The listing builds one solid part. Answer for the finished solid, in the listing's coordinates (mm). A direction names the side the tool comes from. Round coordinates to 2 decimals unless told otherwise and drop trailing zeros. Order: outer loops, then holes, each group sorted by start corner. A loop starts at its lowest first (then second) coordinate and runs counter-clockwise, first axis right, second up. Notation, with made-up numbers: (72, 33) - (88, 33) arc R18 cw to (88, 48) - close; hole circle Ø2 at (60.25, 76.5). An arc over 180 degrees is marked (long way). Use CSV: the item, a comma, the result in double quotes. Start each with the question number.
Item 1: Find section B-B, the plane x = 43.5. Give the vertices of the cut face in (y, z).
Item 2: Flat-ended cylindrical pins translate along their axes: P1, Ø2.5, axis at x = 27.5, z = -15, coming from the +Y side; P2, Ø3.5, axis at x = 28.3, z = -17.12, coming from the -Y side; P3, Ø4, axis at y = 1.5, z = 2.5, coming from the +X side; P4, Ø1.5, axis at y = 2, z = 13.5, coming from the -X side. Find the tip coordinate at first contact, or state that the pin passes through.
Item 3: Find section A-A, the plane y = 4.75. Give the vertices of the cut face in (x, z).
Item 4: Determine the mould class of faces 1 (the flat face through (-49, 3.6, -21)), 2 (the cylindrical face through (42.228, 3.944, -8.156)), 3 (the flat face through (24, 3, 25.135)) for opening direction X: +X half, -X half, draft (parallel to the pull), parting line (faces both ways), or undercut.
Item 5: Straight lines are drawn through the part: line 1 along X through (y, z) = (4.75, -16); line 2 along X through (y, z) = (4.25, -20); line 3 along Z through (x, y) = (48, 5). For each, find the intervals that lie inside material, in ascending order. Write a range as [from, to].
Item 6: For faces 4 (the cylindrical face through (-54.776, 5.818, -19.497)), 5 (the cylindrical face through (24.024, 7.43, 24.534)), determine the directions among +Z, -Z, +X, -X, +Y, -Y from which every point of the face is accessible in a straight line to the end or side of a thin tool.
```python
from build123d import *

# Parameters (mm, degrees)
BOSS_EXTRUDE2_DEPTH                          = 8
CBORE_FOR_M4_HEX_SOCKET_HEAD_CAP_SCR_2_COUNT = 2
CBORE_FOR_M4_HEX_SOCKET_HEAD_CAP_SCR_2_PITCH = 43.312825964
CBORE_FOR_M4_HEX_SOCKET_HEAD_CAP_SCR_3_COUNT = 2
CBORE_FOR_M4_HEX_SOCKET_HEAD_CAP_SCR_3_PITCH = 79.131181871
FILLET1_R                                    = 2


with BuildPart() as part:
    # Sketch6 → Boss-Extrude2 (new body)
    with BuildSketch(Plane(origin=(0, 0, 0), x_dir=(1, 0, 0), z_dir=(0, 1, 0))):
        with BuildLine():
            Line((-49.241489328, 24.864510752), (-56.554028145, 24.864510752))
            ThreePointArc((-56.554028145, 24.864510752), (-41.909367204, -10.490828308), (-6.554028145, -25.135489248))
            Line((-6.554028145, -25.135489248), (55.470114159, -25.135489248))
            Line((55.470114159, -25.135489248), (55.470114159, -6.057055904))
            ThreePointArc((55.470114159, -6.057055904), (42.058086193, 8.373222092), (31.280664632, 24.864510752))
            Line((31.280664632, 24.864510752), (15.257491481, 24.864510752))
            Line((15.257491481, 24.864510752), (-49.241489328, 24.864510752))
        make_face()
    extrude(amount=BOSS_EXTRUDE2_DEPTH)

    # Sketch9 → CBORE for M4 Hex Socket Head Cap Screw1 (revolve, cut)
    with BuildSketch(Plane(origin=(28.299910658, 8, -17.122913845), x_dir=(0, 0, 1), z_dir=(1, 0, 0))):
        Polygon((0, 0), (0, 11.451936393), (2.25, 10.1), (2.25, 4.4), (4, 4.4), (4, 0.025), (4.025, 0), align=None)
    cbore_for_m4_hex_socket_head_cap_screw1 = revolve(axis=Axis((28.299910658, 14.35, -17.122913845), (0, -1, 0)), mode=Mode.SUBTRACT)

    # CBORE for M4 Hex Socket Head Cap Scr 2: CBORE for M4 Hex Socket Head Cap Screw1 ×2
    with Locations(*[Vector(0.5169167622472475, 0, 0.8560356656751065) * (i * CBORE_FOR_M4_HEX_SOCKET_HEAD_CAP_SCR_2_PITCH) for i in range(1, CBORE_FOR_M4_HEX_SOCKET_HEAD_CAP_SCR_2_COUNT)]):
        add(cbore_for_m4_hex_socket_head_cap_screw1, mode=Mode.SUBTRACT)

    # CBORE for M4 Hex Socket Head Cap Scr 3: CBORE for M4 Hex Socket Head Cap Screw1 ×2
    with Locations(*[Vector(-0.9997256378089421, 0, -0.023423259967479314) * (i * CBORE_FOR_M4_HEX_SOCKET_HEAD_CAP_SCR_3_PITCH) for i in range(1, CBORE_FOR_M4_HEX_SOCKET_HEAD_CAP_SCR_3_COUNT)]):
        add(cbore_for_m4_hex_socket_head_cap_screw1, mode=Mode.SUBTRACT)

    # Fillet1
    # the kernel refuses this fillet: 2 mm, written as the material it takes off along each edge
    with BuildSketch(Plane(origin=(-6.554028145, 8, -24.864510752), x_dir=(-0.99500015408545, 0, -0.09987338669500904), z_dir=(0.09987338669500904, 0, -0.99500015408545))) as fillet1_piece_1:
        with BuildLine():
            CenterArc((50 - FILLET1_R, -FILLET1_R), FILLET1_R, 0, 90)
            Line((50, -FILLET1_R), (50, 0))
            Line((50, 0), (50 - FILLET1_R, 0))
        make_face()
    revolve(axis=Axis((-6.554028145, 8, -24.864510752), (0, 1, 0)), revolution_arc=95.731879569, mode=Mode.SUBTRACT)
    with BuildSketch(Plane(origin=(-6.554028145, 8, 25.135489248), x_dir=(0, 0, -1), z_dir=(1, 0, 0))) as fillet1_piece_2:
        with BuildLine():
            CenterArc((FILLET1_R, -FILLET1_R), FILLET1_R, 90, 90)
            Line((0, -FILLET1_R), (0, 0))
            Line((0, 0), (FILLET1_R, 0))
        make_face()
    extrude(amount=67.024142304, mode=Mode.SUBTRACT)


solid = part.part
```
Worked out:
1,outline,"(0, -6.57) - (8, -6.57) - (8, 23.14) arc R2 ccw to (6, 25.14) - (0, 25.14) - close"
2,P1,"stops at y = 3.6"
2,P2,"passes through"
2,P3,"stops at x = 53.79"
2,P4,"stops at x = -39.5"
3,outline,"(-56.55, -24.86) - (31.28, -24.86) arc R116.03 cw to (55.47, 6.06) - (55.47, 25.14) - (-6.55, 25.14) arc R50 ccw to start; hole circle Ø8 at (-50.81, -18.98); hole circle Ø8 at (28.3, -17.12); hole circle Ø8 at (50.69, 19.95)"
4,face 1,"undercut"
4,face 2,"+X half"
4,face 3,"draft"
5,line 1,"x = [-55.76, -53.48], [-48.14, 24.46], [32.14, 36.57]"
5,line 2,"x = [-56.32, -54.68], [-46.94, 25.52], [31.08, 34.05]"
5,line 3,"z = [-1.37, 16.99], [22.92, 25.14]"
6,face 4,"+Y"
6,face 5,"+Z, +X, -X, +Y"
